Autodesk Inventor part; units mm, degrees
ref_plane "Arbeitsebene1" through (0, 0, 65) normal (0, 0, 1) x (1, 0, 0)
ref_plane "YZ Plane" through (0, 0, 0) normal (1, 0, 0) x (0, 1, 0)
ref_plane "XZ Plane" through (0, 0, 0) normal (0, 1, 0) x (-1, 0, 0)
sketch "Skizze1" plane through (0, 0, 0) normal (0, 0, 1) x (1, 0, 0)
  line L0 (0, 0) -> (15, 0)
  line L1 (15, 0) -> (15, 75)
  line L2 (15, 75) -> (0, 75)
  line L3 (0, 75) -> (0, 0)
  dimension "d0" = 15
  dimension "d1" = 75
extrude "Extrusion1" add sketch "Skizze1" along normal blind 130
sketch "Skizze2" plane through (0, 0, 0) normal (-1, 0, 0) x (0, 0, 1)
  line L0 (0, 0) -> (0, 75)
  line L1 (130, 0) -> (130, 75)
  line L2 (0, 33) -> (130, 33)
  line L3 (130, 33) -> (130, 18)
  line L4 (130, 18) -> (0, 18)
  line L5 (0, 18) -> (0, 33)
  line L6 (0, 0) -> (130, 0)
  point P0 (0, 18)
  dimension "d4" = 15
  dimension "d5" = 18
extrude "Extrusion2" add sketch "Skizze2" along normal blind 75 contours L0 L2 L1 L4
ref_plane "Arbeitsebene1" through (0, 0, 65) normal (0, 0, 1) x (1, 0, 0)
sketch "Skizze4" plane through (0, 0, 65) normal (0, 0, 1) x (1, 0, 0)
  line L0 (0, 75) -> (0, 33)
  line L1 (0, 75) -> (-42, 33)
  line L2 (0, 33) -> (-75, 33)
  point P0 (0, 0)
  dimension "d9" = 45
extrude "Extrusion3" add sketch "Skizze4" along normal mid plane 12
sketch "Skizze5" plane through (15, 0, 0) normal (1, 0, 0) x (0, 0, -1)
  line L0 (0, 75) -> (-130, 75)
  line L1 (-87, 75) -> (-75, 75)
  line L2 (-75, 75) -> (-75, 0)
  line L3 (-75, 0) -> (-87, 0)
  line L4 (-87, 0) -> (-87, 75)
  point P0 (0, 0)
  point P1 (-65, 75)
  dimension "d12" = 12
  dimension "d13" = 10
  dimension "d14" = 75
extrude "Extrusion4" add sketch "Skizze5" along normal blind 15
mirror "Spiegeln1" about plane through (0, 0, 65) normal (0, 0, 1) of "Extrusion4"
sketch "Skizze6" plane through (0, 33, 0) normal (-1, 0, 0) x (0, 0, 1)
  line L0 (0, 42) -> (59, 42)
  line L1 (0, 42) -> (0, 0)
  point P0 (0, -33)
  point P1 (20, 12)
  dimension "d24" = 30
  dimension "d25" = 20
hole "Bohrung1" at (0, 45, 20) direction (1, 0, 0) diameter 10 depth 15
sketch "Skizze7" plane through (0, 33, 130) normal (-1, 0, 0) x (0, 0, 1)
  line L0 (0, 0) -> (-130, 0)
  line L1 (0, 42) -> (0, 0)
  point P0 (-130, -33)
  point P1 (-15, 30)
  dimension "d33" = 30
  dimension "d34" = 15
hole "Bohrung" at (0, 63, 115) direction (1, 0, 0) diameter 10 end through all
sketch "Skizze8" plane through (-75, 33, 0) normal (0, 1, 0) x (1, 0, 0)
  line L0 (75, 0) -> (0, 0)
  line L1 (0, -130) -> (0, 0)
  point P0 (15, -15)
  dimension "d42" = 15
  dimension "d43" = 15
hole "Bohrung3" at (-60, 33, 15) direction (0, -1, 0) diameter 16 end through all
sketch "Skizze9" plane through (-75, 33, 0) normal (0, 1, 0) x (1, 0, 0)
  line L0 (75, -130) -> (0, -130)
  line L1 (75, -71) -> (75, -130)
  point P0 (75, 0)
  point P1 (60, -115)
  dimension "d51" = 15
  dimension "d52" = 15
hole "Bohrung4" at (-15, 33, 115) direction (0, -1, 0) diameter 16 end through all
properties part number "lager" material "Edelstahl AISI 202"
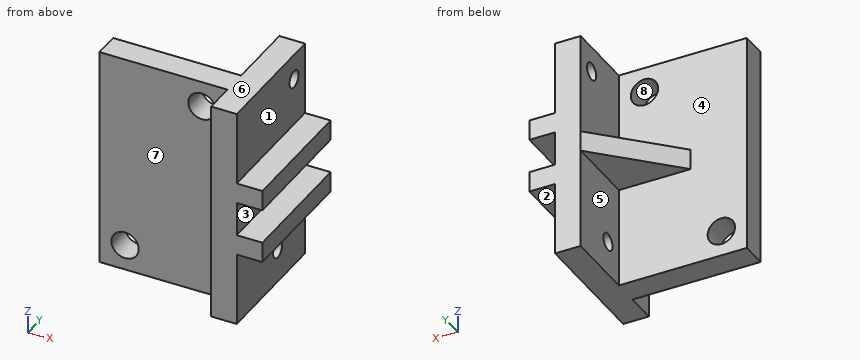
Part model, mm, in its own coordinate system. Face numbers are marked on the shaded views. A direction names the side the tool comes from. Give positions to 0.01 mm unless a question says otherwise; leave off trailing zeros. Write each loop counter-clockwise with the first axis right and the second up, starting at its lowest first coordinate (ties: lowest second). Pieces come first, ordered by that corner, then holes. Notation, with made-up numbers: M 4,32 L 50,32 A15 cw 50,54 Z; hole C 36.25,21 d5. An arc over 180 degrees is marked long. Use CSV: the item, a comma, the result in double quotes.
Item 1: Slice it at A-A on x = -60. Write the cut outline in (y, z), plus the area to 3 significant figures.
Taken from the geometry:
outline,"M 18,0 L 33,0 L 33,7 L 18,7 Z; M 18,23 L 33,23 L 33,130 L 18,130 Z"
area,"1,710 mm²"
Item 2: Pull direction Z, two halves, no side cores. Call the marked faces 6, 7 and 8: +Z half, -Z half, draft (parallel to the pull), parting line (faces both ways), or undercut.
Taken from the geometry:
face 6,"+Z half"
face 7,"draft"
face 8,"undercut"
Item 3: Slice it at C-C on y = 21. Write the cut outline in (x, z).
Taken from the geometry:
outline,"M -75,0 L 15,0 L 15,43 L 30,43 L 30,55 L 15,55 L 15,75 L 30,75 L 30,87 L 15,87 L 15,130 L -75,130 Z; hole C -60,15 d16; hole C -15,115 d16"
Item 4: Drill centre lines: probe 1 along Y at (x, z) = (3, 115); probe 2 along Z at (x, y) = (3.5, 45); probe 3 along Z at (x, y) = (-60, 23). Where is each one in solid material? Low to high.
Taken from the geometry:
probe 1,"y = 0 to 58, 68 to 75"
probe 2,"z = 0 to 15, 25 to 130"
probe 3,"z = 0 to 7, 23 to 130"
Item 5: Pin check, flat tips, straight feed: P1, Ø12, axis at x = 23.5, y = 27.5, coming from the +Z side; P2, Ø8, axis at y = 63, z = 115, coming from the -X side; P3, Ø1, axis at x = -38.5, z = 114, coming from the +Y side; P4, Ø9, axis at y = 6.5, z = 96.5, coming from the -X side. Stop position of each tip, or through.
Taken from the geometry:
P1,"stops at z = 87"
P2,"passes through"
P3,"stops at y = 33"
P4,"stops at x = 0"
Item 6: Slice it at D-D on z = 20. Write the cut outline in (x, y) (3 decimals).
Taken from the geometry:
outline,"M -75,18 L -66.245,18 L -66.245,33 L -75,33 Z; M -53.755,18 L 0,18 L 0,0 L 15,0 L 15,40 L 0,40 L 0,33 L -53.755,33 Z; M 0,50 L 15,50 L 15,75 L 0,75 Z"
Item 7: Slice it at B-B on y = 45. Write the cut outline in (x, z), plus the area to 3 significant figures.
Taken from the geometry:
outline,"M -30,59 L 0,59 L 0,25 L 15,25 L 15,43 L 30,43 L 30,55 L 15,55 L 15,75 L 30,75 L 30,87 L 15,87 L 15,130 L 0,130 L 0,71 L -30,71 Z; M 0,0 L 15,0 L 15,15 L 0,15 Z"
area,"2,520 mm²"
Item 8: Which spindle directions (+Z, -Z, +X, -X, +Y, -Y) get a long thin tool onto all of the face, cutting with end or side? Do the marked faces 1, 2, 3, 4 and 5. Say none if no direction does.
Taken from the geometry:
face 1,"+Z, +X, +Y, -Y"
face 2,"-Z, +X, +Y, -Y"
face 3,"+X, +Y, -Y"
face 4,"-X, +Y"
face 5,"-Z, -X, +Y"
